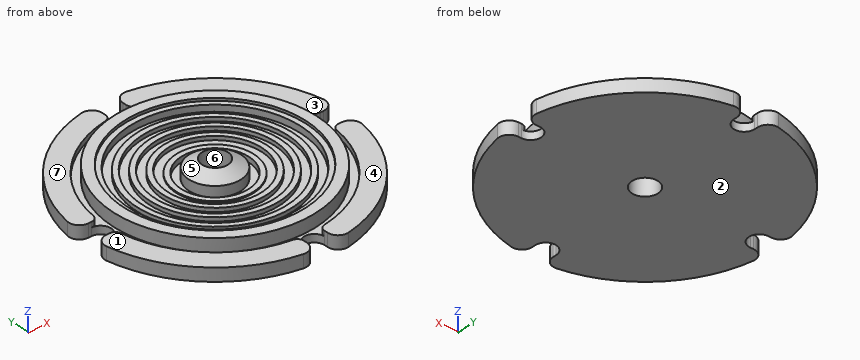
from build123d import *

# Parameters (mm, degrees)
SKETCH_R              = 25
SKETCH_R_2            = 2.5
PAD_DEPTH             = 4
SKETCH001_R           = 25
SKETCH001_R_2         = 19.5
POCKET_DEPTH          = 1.5
SKETCH002_R           = 21
SKETCH002_R_2         = 19.5
POCKET001_DEPTH       = 1
POCKET002_DEPTH       = 5
POLARPATTERN_COUNT    = 4
FILLET_R              = 2
FILLET001_R           = 1.2
SKETCH004_R           = 17.5
POCKET003_DEPTH       = 0.5
SKETCH005_R           = 16.5
SKETCH005_R_2         = 15
POCKET004_DEPTH       = 1.25
SKETCH006_R           = 14
SKETCH006_R_2         = 12.5
POCKET005_DEPTH       = 1.25
SKETCH007_R           = 11.5
SKETCH007_R_2         = 10
POCKET006_DEPTH       = 1.25
SKETCH008_R           = 9
SKETCH008_R_2         = 7.5
POCKET007_DEPTH       = 1.25
SKETCH009_R           = 6.5
SKETCH009_R_2         = 5
POCKET008_DEPTH       = 2
REVOLUTION_FACE59_R   = 15
REVOLUTION_FACE59_R_2 = 14
POCKET009_DEPTH       = 0.5
POCKET009_FACE67_R    = 12.5
POCKET009_FACE67_R_2  = 11.5
POCKET010_DEPTH       = 0.5
POCKET010_FACE64_R    = 10
POCKET010_FACE64_R_2  = 9
POCKET011_DEPTH       = 0.5
POCKET011_FACE56_R    = 7.5
POCKET011_FACE56_R_2  = 6.5
POCKET012_DEPTH       = 0.5
POCKET012_FACE56_R    = 7.5
POCKET012_FACE56_R_2  = 6.5
POCKET013_DEPTH       = 0.5


with BuildPart() as part:
    # Sketch → Pad (new body)
    with BuildSketch(Plane.XY):
        Circle(SKETCH_R)
        Circle(SKETCH_R_2, mode=Mode.SUBTRACT)
    extrude(amount=PAD_DEPTH)

    # Sketch001 (on Face4 of Pad) → Pocket (cut)
    with BuildSketch(Plane.XY.offset(4)):
        Circle(SKETCH001_R)
        Circle(SKETCH001_R_2, mode=Mode.SUBTRACT)
    extrude(amount=-POCKET_DEPTH, mode=Mode.SUBTRACT)

    # Sketch002 (on Face3 of Pocket) → Pocket001 (cut)
    with BuildSketch(Plane.XY.offset(2.5)):
        Circle(SKETCH002_R)
        Circle(SKETCH002_R_2, mode=Mode.SUBTRACT)
    extrude(amount=-POCKET001_DEPTH, mode=Mode.SUBTRACT)

    # Sketch003 (on Face3 of Pocket001) → Pocket002 (cut)
    with BuildSketch(Plane.XY.offset(2.5)):
        with BuildLine():
            Line((22, 2), (27, 2))
            Line((27, 2), (27, -2))
            Line((27, -2), (22, -2))
            ThreePointArc((22, 2), (20, 0), (22, -2))
        make_face()
    pocket002 = extrude(amount=-POCKET002_DEPTH, mode=Mode.SUBTRACT)

    # PolarPattern: Pocket002 ×4 about axis
    polarpattern_axis = Axis((0, 0, 0), (0, 0, 1))
    for i in range(1, POLARPATTERN_COUNT):
        add(pocket002.rotate(polarpattern_axis, i * 360 / POLARPATTERN_COUNT), mode=Mode.SUBTRACT)

    # Fillet
    fillet_edges = [part.edges().sort_by_distance(p)[0] for p in [
        (-2, -24.919872, 1.25),
        (2, -24.919872, 1.25),
        (24.919872, 2, 1.25),
        (24.919872, -2, 1.25),
        (-2, 24.919872, 1.25),
        (2, 24.919872, 1.25),
        (-24.919872, 2, 1.25),
        (-24.919872, -2, 1.25),
    ]]
    fillet(fillet_edges, radius=FILLET_R)

    # Fillet001
    fillet001_edges = [part.edges().sort_by_distance(p)[0] for p in [
        (1.690854, -20.931818, 2),
        (-1.690854, -20.931818, 2),
        (-20.931818, 1.690854, 2),
        (-20.931818, -1.690854, 2),
        (-1.690854, 20.931818, 2),
        (1.690854, 20.931818, 2),
        (20.931818, 1.690854, 2),
        (20.931818, -1.690854, 2),
    ]]
    fillet(fillet001_edges, radius=FILLET001_R)

    # Sketch004 (on Face46 of Fillet001) → Pocket003 (cut)
    with BuildSketch(Plane.XY.offset(4)):
        Circle(SKETCH004_R)
    extrude(amount=-POCKET003_DEPTH, mode=Mode.SUBTRACT)

    # Sketch005 (on Face46 of Pocket003) → Pocket004 (cut)
    with BuildSketch(Plane.XY.offset(3.5)):
        Circle(SKETCH005_R)
        Circle(SKETCH005_R_2, mode=Mode.SUBTRACT)
    extrude(amount=-POCKET004_DEPTH, mode=Mode.SUBTRACT)

    # Sketch006 (on Face46 of Pocket004) → Pocket005 (cut)
    with BuildSketch(Plane.XY.offset(3.5)):
        Circle(SKETCH006_R)
        Circle(SKETCH006_R_2, mode=Mode.SUBTRACT)
    extrude(amount=-POCKET005_DEPTH, mode=Mode.SUBTRACT)

    # Sketch007 (on Face46 of Pocket005) → Pocket006 (cut)
    with BuildSketch(Plane.XY.offset(3.5)):
        Circle(SKETCH007_R)
        Circle(SKETCH007_R_2, mode=Mode.SUBTRACT)
    extrude(amount=-POCKET006_DEPTH, mode=Mode.SUBTRACT)

    # Sketch008 (on Face46 of Pocket006) → Pocket007 (cut)
    with BuildSketch(Plane.XY.offset(3.5)):
        Circle(SKETCH008_R)
        Circle(SKETCH008_R_2, mode=Mode.SUBTRACT)
    extrude(amount=-POCKET007_DEPTH, mode=Mode.SUBTRACT)

    # Sketch009 (on Face46 of Pocket007) → Pocket008 (cut)
    with BuildSketch(Plane.XY.offset(3.5)):
        Circle(SKETCH009_R)
        Circle(SKETCH009_R_2, mode=Mode.SUBTRACT)
    extrude(amount=-POCKET008_DEPTH, mode=Mode.SUBTRACT)

    # Sketch010 → Revolution (revolve)
    with BuildSketch(Plane.XZ):
        Polygon((2.5, 3.5), (5, 3.5), (2.5, 5), align=None)
    revolve(axis=Axis((0, 0, 0), (0, 0, 1)))

    # Revolution Face59 → Pocket009 (cut)
    with BuildSketch(Plane(origin=(0, 0, 3.5), x_dir=(0, 1, 0), z_dir=(0, 0, 1))):
        Circle(REVOLUTION_FACE59_R)
        Circle(REVOLUTION_FACE59_R_2, mode=Mode.SUBTRACT)
    extrude(amount=-POCKET009_DEPTH, mode=Mode.SUBTRACT)

    # Pocket009 Face67 → Pocket010 (cut)
    with BuildSketch(Plane(origin=(0, 0, 3.5), x_dir=(0, 1, 0), z_dir=(0, 0, 1))):
        Circle(POCKET009_FACE67_R)
        Circle(POCKET009_FACE67_R_2, mode=Mode.SUBTRACT)
    extrude(amount=-POCKET010_DEPTH, mode=Mode.SUBTRACT)

    # Pocket010 Face64 → Pocket011 (cut)
    with BuildSketch(Plane(origin=(0, 0, 3.5), x_dir=(0, 1, 0), z_dir=(0, 0, 1))):
        Circle(POCKET010_FACE64_R)
        Circle(POCKET010_FACE64_R_2, mode=Mode.SUBTRACT)
    extrude(amount=-POCKET011_DEPTH, mode=Mode.SUBTRACT)

    # Pocket011 Face56 → Pocket012 (cut)
    with BuildSketch(Plane(origin=(0, 0, 3.5), x_dir=(0, 1, 0), z_dir=(0, 0, 1))):
        Circle(POCKET011_FACE56_R)
        Circle(POCKET011_FACE56_R_2, mode=Mode.SUBTRACT)
    extrude(amount=-POCKET012_DEPTH, mode=Mode.SUBTRACT)

    # Pocket012 Face56 → Pocket013 (cut)
    with BuildSketch(Plane(origin=(0, 0, 3), x_dir=(0, 1, 0), z_dir=(0, 0, 1))):
        Circle(POCKET012_FACE56_R)
        Circle(POCKET012_FACE56_R_2, mode=Mode.SUBTRACT)
    extrude(amount=-POCKET013_DEPTH, mode=Mode.SUBTRACT)


solid = part.part
CAD build for the part. Positions are in the model's coordinates, mm. Face numbers are marked on the shaded views. A direction names the side the tool comes from. Round coordinates to 2 decimals unless told otherwise and drop trailing zeros. Use a Markdown table: item, result. Add a question column.
1. Pull direction Y, two halves, no side cores. Call the marked faces 6 and 7: released by +Y, released by -Y, zero draft, split by the parting line, or undercut.
2. Flat gauge pins, fed straight in: P1, Ø3, axis at y = 17, z = 4.5, coming from the +X side; P2, Ø0.7, axis at x = 22, z = 1.5, coming from the -Y side; P3, Ø6, axis at x = -2, y = 0, coming from the +Z side; P4, Ø0.7, axis at x = -22.5, z = 0.5, coming from the -Y side. Where does each tip first touch, or does it go through?
3. Drill centre lines: probe 1 along Y at (x, z) = (0, 2); probe 2 along Y at (x, z) = (0, 3.2); probe 3 along Y at (x, z) = (0, 1.25). Where is each one in solid material? Low to high.
4. 3-axis set-ups, long thin cutter, end or side, ignore diameter. For the marked faces 1, 2, 3, 4 and 5: which of +Z, -Z, +X, -X, +Y, -Y reach the whole face in a straight line?
Reply:
| question | item | result |
|---|---|---|
| 1 | face 6 | undercut |
| 1 | face 7 | zero draft |
| 2 | P1 | stops at x = 11.72 |
| 2 | P2 | stops at y = -12.5 |
| 2 | P3 | stops at z = 5 |
| 2 | P4 | stops at y = -11.59 |
| 3 | probe 1 | y = -19.5 to -6.5, -5 to -2.5, 2.5 to 5, 6.5 to 19.5 |
| 3 | probe 2 | y = -19.5 to -16.5, -5 to -2.5, 2.5 to 5, 16.5 to 19.5 |
| 3 | probe 3 | y = -20 to -2.5, 2.5 to 20 |
| 4 | face 1 | +Z, -X, -Y |
| 4 | face 2 | -Z, +X, -X, +Y, -Y |
| 4 | face 3 | +Z, +X, +Y |
| 4 | face 4 | +Z, +X, -Y |
| 4 | face 5 | +Z |
